Here's how the part is built. I have some questions about the finished solid (model axes, mm). A direction names the side the tool comes from. Coordinates: 2 decimals unless noted, no trailing zeros. Write each loop counter-clockwise with the first axis right and the second up, starting at its lowest first coordinate (ties: lowest second). Pieces come first, ordered by that corner, then holes.
```python
from build123d import *

# Parameters (mm, degrees)
F0_R     = 4.180396
F1_DEPTH = 3.96875


with BuildPart() as f1:
    # F0 (on Front) → F1 (new body, symmetric)
    with BuildSketch(Plane.XZ):
        with BuildLine():
            ThreePointArc((0, -19.2024), (-19.2024, 0), (0, 19.2024))
            Line((0, 19.2024), (0, 30.226))
            Line((0, 30.226), (-17.022172, 30.226))
            Line((-17.022172, 30.226), (-17.022172, 24.332866))
            ThreePointArc((-17.022172, 24.332866), (-17.323239, 22.983372), (-18.169343, 21.889808))
            ThreePointArc((-18.169343, 21.889808), (-22.721865, 17.117405), (-26.05303, 11.4249))
            ThreePointArc((-26.05303, 11.4249), (-27.224045, 10.042081), (-28.960734, 9.525))
            Line((-28.960734, 9.525), (-136.386337, 9.525))
            ThreePointArc((-136.386337, 9.525), (-139.561337, 8.674261), (-141.885599, 6.35))
            Line((-141.885599, 6.35), (-165.349114, -34.29))
            ThreePointArc((-165.349114, -34.29), (-162.56, -44.699114), (-152.150886, -41.91))
            Line((-152.150886, -41.91), (-134.380152, -11.113158))
            ThreePointArc((-134.380152, -11.113158), (-133.217971, -9.950559), (-131.630142, -9.525))
            Line((-131.630142, -9.525), (-28.960734, -9.525))
            ThreePointArc((-28.960734, -9.525), (-27.224045, -10.042081), (-26.05303, -11.4249))
            ThreePointArc((-26.05303, -11.4249), (-23.2839, -16.344684), (-19.597776, -20.620763))
            ThreePointArc((-19.597776, -20.620763), (-18.884031, -21.631899), (-18.611115, -22.839104))
            Line((-18.611115, -22.839104), (-18.417747, -30.226))
            Line((-18.417747, -30.226), (0, -30.226))
            Line((0, -30.226), (0, -19.2024))
        make_face()
        with Locations((-158.75, -38.1)):
            Circle(F0_R, mode=Mode.SUBTRACT)
    extrude(amount=F1_DEPTH, both=True)


solid = f1.part
```
1) We'd pull the mould along Z, two halves only. Please class faces 1 (the face through (0, 0, 25)), 2 (the face through (-153.453, -0.056, -13.686)), 3 (the face through (-19.2, -0.1, -0.4)): pulls with the +Z half, pulls with the -Z half, needs draft (parallel to the pull), parting line crosses it, or undercut.
Values follow:
face 1: needs draft
face 2: pulls with the +Z half
face 3: undercut
2) Imagine slicing it at B-B on x = -158.75. Please give me the cut outline in (y, z).
Values follow:
outline: (-3.97, -45.72) - (3.97, -45.72) - (3.97, -42.28) - (-3.97, -42.28) - close; (-3.97, -33.92) - (3.97, -33.92) - (3.97, -22.86) - (-3.97, -22.86) - close
3) On a 3-axis mill with a long thin cutter (end or side, diameter ignored), from which of +Z, -Z, +X, -X, +Y, -Y can I reach the whole of each face in a straight line? I mean faces 4 (the face through (-133.238, -0.056, -9.962)), 5 (the face through (-17.022, 0, 27)), 6 (the face through (-9, 0, -30.226)). Say none if no direction works.
Values follow:
face 4: -Z, +Y, -Y
face 5: +Z, -X, +Y, -Y
face 6: -Z, +X, +Y, -Y
4) I need wall thicknesses on probe 1 along Z at (x, y) = (-30, 2.5) (3 decimals); probe 2 along X at (y, z) = (3.75, 26); probe 3 along X at (y, z) = (-3, -27.5). Which ranges of each line are inside material? Lowest first, please.
Values follow:
probe 1: z = -9.525 to 9.525
probe 2: x = -17.02 to 0
probe 3: x = -161.43 to -143.84, -18.49 to 0
5) Will these pins go through, and if not, where does the flat tip stop? pin 1 (4 mm diameter, centred on x = -132, y = -1, fed in from -Z); pin 2 (2 mm diameter, centred on x = -88, y = -1, fed in from -Z) (3 decimals); pin 3 (2.5 mm diameter, centred on x = -97, y = 1, fed in from +Z) (3 decimals).
Values follow:
pin 1: stops at z = -10.59
pin 2: stops at z = -9.525
pin 3: stops at z = 9.525
6) Imagine slicing it at C-C on z = -38.1. Please give me the cut outline in (x, y), then the cut area to 3 significant figures.
Values follow:
outline: (-166.37, -3.97) - (-162.93, -3.97) - (-162.93, 3.97) - (-166.37, 3.97) - close; (-154.57, -3.97) - (-149.95, -3.97) - (-149.95, 3.97) - (-154.57, 3.97) - close
area: 64.0 mm2
7) Imagine slicing it at D-D on x = -110. Please give me the cut outline in (y, z) (3 decimals), then the cut area to 3 significant figures.
Values follow:
outline: (-3.969, -9.525) - (3.969, -9.525) - (3.969, 9.525) - (-3.969, 9.525) - close
area: 151 mm2
8) Imagine slicing it at A-A on y = -2. Please give me the cut outline in (x, z) (3 decimals).
Values follow:
outline: (-165.349, -34.29) arc R7.62 ccw to (-152.151, -41.91) - (-134.38, -11.113) arc R3.175 cw to (-131.63, -9.525) - (-28.961, -9.525) arc R3.175 cw to (-26.053, -11.425) arc R28.448 ccw to (-19.598, -20.621) arc R3.175 cw to (-18.611, -22.839) - (-18.418, -30.226) - (0, -30.226) - (0, -19.202) arc R19.202 cw to (0, 19.202) - (0, 30.226) - (-17.022, 30.226) - (-17.022, 24.333) arc R3.175 cw to (-18.169, 21.89) arc R28.448 ccw to (-26.053, 11.425) arc R3.175 cw to (-28.961, 9.525) - (-136.386, 9.525) arc R6.35 ccw to (-141.886, 6.35) - close; hole circle Ø8.361 at (-158.75, -38.1)
